Source: three-view drawing plus pictorial views. Frame: mm from the lowest corner of the part. Coordinates: 2 decimals unless noted, no trailing zeros. Write each loop counter-clockwise with the first axis right and the second up, starting at its lowest first coordinate (ties: lowest second). Pieces come first, ordered by that corner, then holes. Notation, with made-up numbers: M -36,49 L 15,49 A7 ccw 15,58 Z; hole C 30.25,80.25 d8. An arc over 180 degrees is marked long. Use CSV: the item, a comma, the result in double quotes.
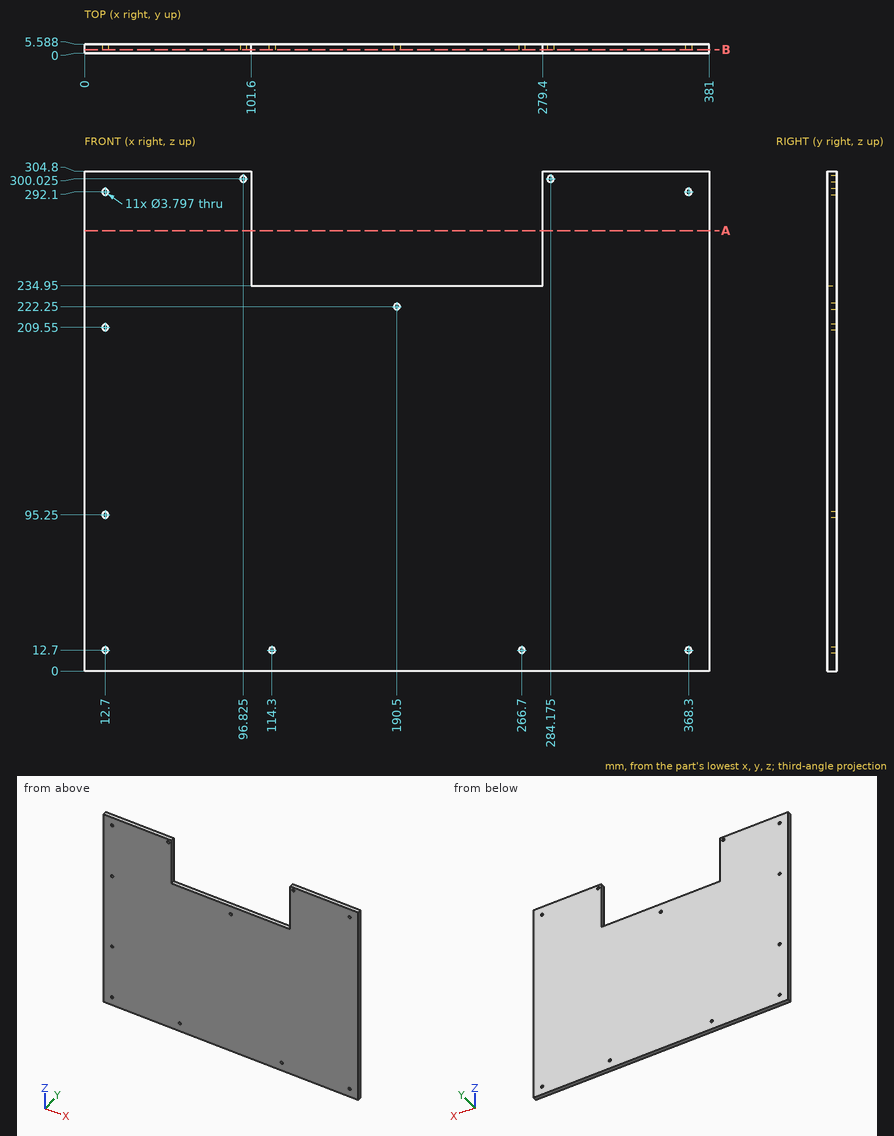
1. Contact query for a flat-ended pin moving along its axis: pin 1 Ø3 at (x, y) = (194.5, 3) entering from +Z. Output: stop coordinate, or through.
Resolved:
pin 1,"stops at z = 234.95"
2. Section A-A (z = 268.5). Return loops of the section in (x, y), then the cut area to 3 significant figures.
Resolved:
outline,"M 0,0 L 101.6,0 L 101.6,5.59 L 0,5.59 Z; M 279.4,0 L 381,0 L 381,5.59 L 279.4,5.59 Z"
area,"1,140 mm^2"
3. Section B-B (y = 2.1). State how many separate pieces and enclosed holes the cut face has, then the cut area to 3 significant figures.
Resolved:
separate pieces,"1"
enclosed holes,"11"
area,"104,000 mm^2"
4. Material intervals for line 1 (X direction, y = 2, z = 12.7); line 2 (Z direction, x = 12.7, y = 3.7); line 3 (X direction, y = 1.5, z = 292.1), sorted ascending. Write a range as [from, to].
Resolved:
line 1,"x = [0, 10.8], [14.6, 112.4], [116.2, 264.8], [268.6, 366.4], [370.2, 381]"
line 2,"z = [0, 10.8], [14.6, 93.35], [97.15, 207.65], [211.45, 290.2], [294, 304.8]"
line 3,"x = [0, 10.8], [14.6, 101.6], [279.4, 366.4], [370.2, 381]"
